Source: three-view drawing plus pictorial views. Frame: mm from the lowest corner of the part. Give positions to 0.01 mm unless a question says otherwise; leave off trailing zeros. Loops run counter-clockwise (first coordinate to the right, second up) from the corner with the lowest first, then second, coordinate; pieces in that order, holes last. Notation, with made-up numbers: (53.25, 46.5) - (72.25, 46.5) arc R23 ccw to (72.25, 67.5) - close; hole circle Ø5 at (-37, 80.25). An arc over 180 degrees is marked (long way). Write each question's results on one line, items separated by ' | '. Start each with the question number.
(1) Contact query for a flat-ended pin moving along its axis: pin 1 (6 mm diameter, centred on x = 118.5, z = 11.5, fed in from +Y). Output: stop coordinate, or through.
(2) Cut plane C-C on x = 86. Return the cut outline in (y, z).
(3) Cut plane A-A on y = 56. Return the cut outline in (x, z).
(4) Pull-direction query (Y, two-part tool) for the marked faces 1, 2 and 3; classes: pulls with the +Y half, pulls with the -Y half, needs draft (parallel to the pull), parting line crosses it, or undercut.
(5) Cut plane D-D on z = 18.5. Return the cut outline in (x, y).
(6) Cut plane B-B on z = 10. Return the cut outline in (x, y).
(7) Material intervals for line 1 along X through (y, z) = (49, 10); line 2 along Z through (x, y) = (145, 25.5); line 3 along X through (y, z) = (55.5, 5.5), sorted ascending. Write a range as [from, to].
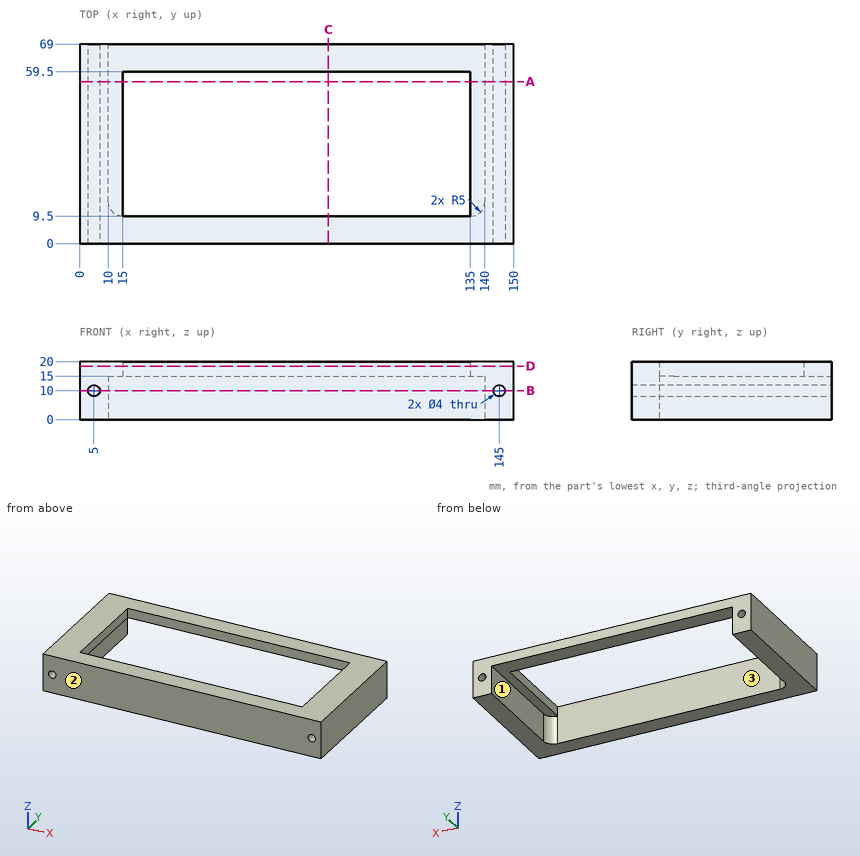
Ans:
1) pin 1: y = 9.5
2) outline: (0, 0) - (9.5, 0) - (9.5, 20) - (0, 20) - close; (59.5, 15) - (69, 15) - (69, 20) - (59.5, 20) - close
3) outline: (0, 0) - (10, 0) - (10, 15) - (15, 15) - (15, 20) - (0, 20) - close; (135, 15) - (140, 15) - (140, 0) - (150, 0) - (150, 20) - (135, 20) - close; hole circle Ø4 at (5, 10); hole circle Ø4 at (145, 10)
4) face 1: needs draft | face 2: pulls with the -Y half | face 3: undercut
5) outline: (0, 0) - (150, 0) - (150, 69) - (0, 69) - close; hole (15, 9.5) - (135, 9.5) - (135, 59.5) - (15, 59.5) - close
6) outline: (0, 0) - (3, 0) - (3, 69) - (0, 69) - close; (7, 0) - (143, 0) - (143, 69) - (140, 69) - (140, 14.5) arc R5 cw to (135, 9.5) - (15, 9.5) arc R5 cw to (10, 14.5) - (10, 69) - (7, 69) - close; (147, 0) - (150, 0) - (150, 69) - (147, 69) - close
7) line 1: [0, 3], [7, 10], [140, 143], [147, 150] | line 2: [0, 8], [12, 20] | line 3: [0, 10], [140, 150]
